Here's how the part is built. I have some questions about the finished solid (model axes, mm). Face numbers are marked on the shaded views. A direction names the side the tool comes from. Coordinates: 2 decimals unless noted, no trailing zeros. Write each loop counter-clockwise with the first axis right and the second up, starting at its lowest first coordinate (ties: lowest second). Pieces come first, ordered by that corner, then holes. Notation, with made-up numbers: (-35, 15) -> (-26, 15) arc R27 cw to (-26, 54) -> close; hole circle Ø5 at (51.5, 37). An arc over 180 degrees is marked (long way). Answer in a Markdown table with one row per item. Add a question column.
from build123d import *

# Parameters (mm, degrees)
ESQUISSE1_W             = 90
ESQUISSE1_H             = 40
BOSS_EXTRU_1_DEPTH      = 12
ESQUISSE2_R             = 4
ENL_V_MAT_EXTRU_1_DEPTH = 62.392181913
ESQUISSE3_R             = 7.75
ENL_V_MAT_EXTRU_2_DEPTH = 12.25
ESQUISSE9_W             = 50
ESQUISSE9_H             = 14.72812859
ESQUISSE9_H_2           = 10.600161614
ENL_V_MAT_EXTRU_7_DEPTH = 31
BOSS_EXTRUDE1_DEPTH     = 5
SKETCH2_R               = 2.1
CUT_EXTRUDE1_DEPTH      = 53.096065111
SKETCH3_R               = 4
CUT_EXTRUDE2_DEPTH      = 10
CUT_EXTRUDE3_DEPTH      = 5
SKETCH6_W               = 4
SKETCH6_H               = 31
SKETCH7_W               = 1.5
SKETCH7_H               = 10.5
SKETCH7_H_2             = 4
SKETCH7_W_2             = 5.75
SKETCH7_H_3             = 1.5
BOSS_EXTRUDE2_START     = 4.5
BOSS_EXTRUDE2_DEPTH     = 4.5
BOSS_EXTRUDE3_DEPTH     = 4.5


with BuildPart() as part:
    # Esquisse1 → Boss.-Extru.1 (new body)
    with BuildSketch(Plane.XY):
        Rectangle(ESQUISSE1_W, ESQUISSE1_H)
    extrude(amount=BOSS_EXTRU_1_DEPTH)

    # Esquisse2 → Enl_v. mat.-Extru.1 (cut, through all)
    with BuildSketch(Plane(origin=(0, 20, 0), x_dir=(1, 0, 0), z_dir=(0, 1, 0))):
        with Locations((-30, -12)):
            Circle(ESQUISSE2_R)
        with Locations((30, -12)):
            Circle(ESQUISSE2_R)
    extrude(amount=-ENL_V_MAT_EXTRU_1_DEPTH, mode=Mode.SUBTRACT)

    # Esquisse3 → Enl_v. mat.-Extru.2 (cut, symmetric)
    with BuildSketch(Plane(origin=(0, 0, 0), x_dir=(1, 0, 0), z_dir=(0, 1, 0))):
        with Locations((-30, -12)):
            Circle(ESQUISSE3_R)
    enl_v_mat_extru_2 = extrude(amount=ENL_V_MAT_EXTRU_2_DEPTH, both=True, mode=Mode.SUBTRACT)

    # Esquisse9 → Enl_v. mat.-Extru.7 (cut)
    with BuildSketch(Plane.XY.offset(12)):
        with Locations((0, -22.864064295)):
            Rectangle(ESQUISSE9_W, ESQUISSE9_H)
        with Locations((0, 20.800080807)):
            Rectangle(ESQUISSE9_W, ESQUISSE9_H_2)
    extrude(amount=-ENL_V_MAT_EXTRU_7_DEPTH, mode=Mode.SUBTRACT)

    # Sketch1 → Boss-Extrude1 (add)
    with BuildSketch(Plane(origin=(0, 0, 0), x_dir=(-1, 0, 0), z_dir=(0, 0, -1))):
        Polygon((-25, -15.5), (25, -15.5), (25, -20), (45, -20), (45, 20), (25, 20), (25, 15.5), (-25, 15.5), (-25, 20), (-45, 20), (-45, -20), (-25, -20), align=None)
    extrude(amount=BOSS_EXTRUDE1_DEPTH)

    # Sketch2 → Cut-Extrude1 (cut, through all)
    with BuildSketch(Plane.XY.offset(12)):
        with Locations((-40, 10.5)):
            Circle(SKETCH2_R)
        with Locations(Location((40, 10.5, 0), (0, 0, 180))):
            Circle(SKETCH2_R)
        with Locations((40, -10.5)):
            Circle(SKETCH2_R)
        with Locations(Location((-40, -10.5, 0), (0, 0, 180))):
            Circle(SKETCH2_R)
    extrude(amount=-CUT_EXTRUDE1_DEPTH, mode=Mode.SUBTRACT)

    # Sketch3 → Cut-Extrude2 (cut)
    with BuildSketch(Plane(origin=(0, 0, -5), x_dir=(-1, 0, 0), z_dir=(0, 0, -1))):
        with Locations((-40, 10.5)):
            Circle(SKETCH3_R)
        with Locations((40, 10.5)):
            Circle(SKETCH3_R)
        with Locations((40, -10.5)):
            Circle(SKETCH3_R)
        with Locations((-40, -10.5)):
            Circle(SKETCH3_R)
    extrude(amount=-CUT_EXTRUDE2_DEPTH, mode=Mode.SUBTRACT)

    # Sketch4 → Cut-Extrude3 (cut)
    with BuildSketch(Plane(origin=(0, 0, -5), x_dir=(-1, 0, 0), z_dir=(0, 0, -1))):
        with BuildLine():
            Line((-36, 10.5), (-36, 20))
            Line((-36, 20), (-45, 20))
            Line((-45, 20), (-45, 6.5))
            Line((-45, 6.5), (-40, 6.5))
            ThreePointArc((-40, 6.5), (-42.828427125, 13.328427125), (-36, 10.5))
        make_face()
        with BuildLine():
            Line((-40, -6.5), (-50, -6.5))
            Line((-50, -6.5), (-45, -20))
            Line((-45, -20), (-36, -20))
            Line((-36, -20), (-36, -10.5))
            ThreePointArc((-36, -10.5), (-42.828427125, -13.328427125), (-40, -6.5))
        make_face()
        with BuildLine():
            Line((45, -20), (45, -6.5))
            Line((45, -6.5), (40, -6.5))
            ThreePointArc((40, -6.5), (42.828427125, -13.328427125), (36, -10.5))
            Line((36, -10.5), (36, -20))
            Line((36, -20), (45, -20))
        make_face()
        with BuildLine():
            Line((40, 6.5), (45, 6.5))
            Line((45, 6.5), (45, 20))
            Line((45, 20), (36, 20))
            Line((36, 20), (36, 10.5))
            ThreePointArc((36, 10.5), (42.828427125, 13.328427125), (40, 6.5))
        make_face()
    extrude(amount=-CUT_EXTRUDE3_DEPTH, mode=Mode.SUBTRACT)

    # Mirror1: Enl_v. mat.-Extru.2 across plane
    add(enl_v_mat_extru_2.mirror(Plane.ZY), mode=Mode.SUBTRACT)

    # Sketch6 → Cut-Revolve1 (revolve, cut)
    with BuildSketch(Plane.XY.offset(12)):
        with Locations((-2, 0)):
            Rectangle(SKETCH6_W, SKETCH6_H)
    revolve(axis=Axis((0, -15.5, 12), (0, 1, 0)), mode=Mode.SUBTRACT)

    # Sketch7 → Cut-Revolve4 (revolve, cut)
    with BuildSketch(Plane.XY.offset(12)):
        with Locations((-4.75, 2.75)):
            Rectangle(SKETCH7_W, SKETCH7_H)
        with Locations((-4.75, -4.5)):
            Rectangle(SKETCH7_W, SKETCH7_H_2)
        with Locations((-8.375, -4.5)):
            Rectangle(SKETCH7_W_2, SKETCH7_H_2)
        with Locations((-4.75, -7.25)):
            Rectangle(SKETCH7_W, SKETCH7_H_3)
    revolve(axis=Axis((0, 8, 12), (0, -1, 0)), mode=Mode.SUBTRACT)

    # Sketch8 → Boss-Extrude2 (add)
    with BuildSketch(Plane(origin=(0, 15.5, 0), x_dir=(1, 0, 0), z_dir=(0, 1, 0)).offset(BOSS_EXTRUDE2_START)):
        with BuildLine():
            Line((4, -12), (25, -12))
            Line((25, -12), (25, 5))
            Line((25, 5), (-25, 5))
            Line((-25, 5), (-25, -12))
            Line((-25, -12), (-4, -12))
            ThreePointArc((-4, -12), (0, -8), (4, -12))
        make_face()
    extrude(amount=-BOSS_EXTRUDE2_DEPTH)

    # Sketch9 → Boss-Extrude3 (add)
    with BuildSketch(Plane.XZ.offset(15.5)):
        with BuildLine():
            Line((-4, 12), (-25, 12))
            Line((-25, 12), (-25, -5))
            Line((-25, -5), (25, -5))
            Line((25, -5), (25, 12))
            Line((25, 12), (4, 12))
            ThreePointArc((4, 12), (0, 8), (-4, 12))
        make_face()
    extrude(amount=BOSS_EXTRUDE3_DEPTH)


solid = part.part
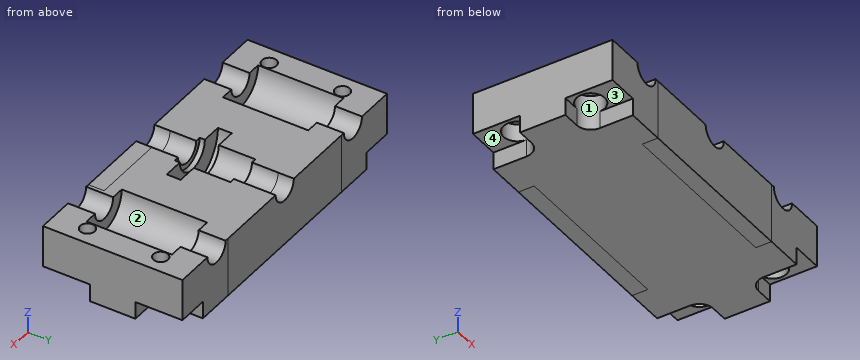
Q1. Imagine slicing it at D-D on z = -2.25. Please give me the cut outline in (x, y).
Q2. Imagine slicing it at A-A on x = 0. Please give me the cut outline in (y, z).
Q3. Imagine slicing it at B-B on z = 3. Please give me the cut outline in (x, y), plus the area to 3 significant figures.
Q4. I'm going to push flat-ended pins straight in: P1, Ø4, axis at x = 40, y = -10.5, coming from the -Z side; P2, Ø2.5, axis at x = 38, y = -11.5, coming from the -Z side; P3, Ø1.5, axis at y = -16.5, z = -2.5, coming from the +X side; P4, Ø4.5, axis at x = -40.5, y = -16.5, coming from the -Z side. Where does each tip first touch, or does it pass through?
Q5. Imagine slicing it at C-C on y = -5.5. Please give me the cut outline in (x, z).
Q6. For the marked faces 1, 2, 3 and 4, which set-ups out of +Z, -Z, +X, -X, +Y, -Y let a thin tool reach every point of the face, with its end or its side?
Q7. I need wall thicknesses on line 1 (X direction, y = 10.5, z = 0.5); line 2 (Y direction, x = 40, z = 9.75); line 3 (Y direction, x = -25.5, z = 7). Which ranges of each line are inside material? Lowest first, please. Write a range as [from, to].
Result sheet:
| question | item | result |
|---|---|---|
| 1 | outline | (-45, -6.5) -> (-40, -6.5) arc R4 cw to (-36, -10.5) -> (-36, -20) -> (36, -20) -> (36, -10.5) arc R4 cw to (40, -6.5) -> (45, -6.5) -> (45, 6.5) -> (40, 6.5) arc R4 cw to (36, 10.5) -> (36, 20) -> (-36, 20) -> (-36, 10.5) arc R4 cw to (-40, 6.5) -> (-45, 6.5) -> close |
| 2 | outline | (-20, -5) -> (20, -5) -> (20, 8) -> (8, 8) -> (8, 6.5) -> (-2.5, 6.5) -> (-2.5, 0.75) -> (-6.5, 0.75) -> (-6.5, 6.5) -> (-8, 6.5) -> (-8, 8) -> (-20, 8) -> close |
| 3 | outline | (-45, -20) -> (45, -20) -> (45, 20) -> (-45, 20) -> close; hole circle Ø8 at (-40, -10.5); hole circle Ø8 at (-40, 10.5); hole (-6.75, -6.5) -> (6.75, -6.5) -> (6.75, -2.5) -> (-6.75, -2.5) -> close; hole circle Ø8 at (40, -10.5); hole circle Ø8 at (40, 10.5) |
| 3 | area | 3,340 mm^2 |
| 4 | P1 | passes through |
| 4 | P2 | stops at z = 5 |
| 4 | P3 | stops at x = 36 |
| 4 | P4 | stops at z = 0 |
| 5 | outline | (-45, -5) -> (45, -5) -> (45, 12) -> (37.75, 12) arc R7.75 cw to (22.25, 12) -> (11.25, 12) arc R11.25 cw to (-11.25, 12) -> (-22.25, 12) arc R7.75 cw to (-37.75, 12) -> (-45, 12) -> close |
| 6 | face 1 | -Z |
| 6 | face 2 | +Z |
| 6 | face 3 | -Z, -X, -Y |
| 6 | face 4 | -Z, -X, +Y |
| 7 | line 1 | x = [-45, -44], [-36, 36], [44, 45] |
| 7 | line 2 | y = [-20, -12.6], [-8.4, 8.4], [12.6, 20] |
| 7 | line 3 | y = [-20, -12.25], [12.25, 20] |
